Here's how the part is built. I have some questions about the finished solid (model axes, mm). Face numbers are marked on the shaded views. A direction names the side the tool comes from. Round coordinates to 2 decimals unless told otherwise and drop trailing zeros. Write each loop counter-clockwise with the first axis right and the second up, starting at its lowest first coordinate (ties: lowest second). Pieces come first, ordered by that corner, then holes. Notation, with made-up numbers: (85.5, 64) -> (97.5, 64) arc R18 ccw to (97.5, 87) -> close; hole circle Ø9 at (32.5, 4). An arc over 180 degrees is marked (long way). Put each result on its own line as item: value. Start each with the question number.
1) I want a section at A-A, the plane y = 16.5. List the corners of the cut face in (x, z) for me, then the cut area to 3 significant figures.
2) I want a section at C-C, the plane x = 10.5. List the corners of the cut face in (y, z) for me, then the cut area to 3 significant figures.
3) I want a section at D-D, the plane z = 4.75. List the corners of the cut face in (x, y) for me.
4) Will these pins go through, and if not, where does the flat tip stop? P1, Ø0.6, axis at y = 3, z = 10.5, coming from the +X side; P2, Ø3, axis at x = 34, z = 8.5, coming from the -Y side; P3, Ø8, axis at x = 36, y = 10, coming from the +Z side; P4, Ø4, axis at x = 19.5, y = 5, coming from the +Z side.
5) We'd pull the mould along Z, two halves only. Please class the marked faces 4, 5 and 6: released by +Z, released by -Z, zero draft, split by the parting line, or undercut.
6) If I drill on line 1 along Y through (x, z) = (22, 0.2); line 2 along Z through (x, y) = (23, 31.5); line 3 along Z through (x, y) = (24, 13), over which ranges is the centre line in solid material (lowest first)? Write a range as [from, to].
7) I want a section at B-B, the plane x = 33. List the corners of the cut face in (y, z) for me, then the cut area to 3 significant figures.
8) Which directions (+Z, -Z, +X, -X, +Y, -Y) give clear straight access to the entire face, cutting with the end or side of a thin tool? Please do the marked faces 1, 2 and 3.
Autodesk Inventor part; units mm, degrees
ref_plane "YZ Plane" through (0, 0, 0) normal (1, 0, 0) x (0, 1, 0)
ref_plane "XZ Plane" through (0, 0, 0) normal (0, 1, 0) x (-1, 0, 0)
ref_plane "XY Plane" through (0, 0, 0) normal (0, 0, 1) x (1, 0, 0)
sketch "Sketch1" plane through (0, 0, 0) normal (0, 0, 1) x (1, 0, 0)
  line L0 (0, 0) -> (44, 0)
  line L1 (44, 0) -> (44, 33)
  line L2 (44, 33) -> (0, 33)
  line L3 (0, 33) -> (0, 0)
  line L4 (2, 1.5) -> (44, 1.5)
  line L5 (44, 1.5) -> (44, 31.5)
  line L6 (44, 31.5) -> (2, 31.5)
  line L7 (2, 31.5) -> (2, 1.5)
  dimension "d0" = 44
  dimension "d1" = 33
  dimension "d2" = 42
  dimension "d3" = 30
  dimension "d4" = 2
  dimension "d5" = 0
  dimension "d6" = 1.5
extrude "Extrusion1" add sketch "Sketch1" along normal blind 11
shell "Shell1" thickness 1.25 removed faces 1 at (44, 11, 3.6667)
sketch "Sketch2" plane through (0, 0, 11) normal (0, 0, 1) x (1, 0, 0)
  circle A0 centre (22, 16.5) radius 8
  circle A1 centre (22, 16.5) radius 8.75
  point P0 (0, 0)
  dimension "d10" = 16
  dimension "d11" = 17.5
extrude "Extrusion2" add sketch "Sketch2" along normal blind 1.5
sketch "Sketch3" plane through (22, 16.5, 11) normal (0, 0, 1) x (1, 0, 0)
  line L0 (1.47, 5.1769) -> (11.6334, 5.1769)
  line L1 (11.6334, 5.1769) -> (11.6334, -5.2059)
  line L2 (11.6334, -5.2059) -> (1.47, -5.2059)
  line L3 (1.47, -5.2059) -> (1.47, 5.1769)
  line L4 (1.47, 5.1769) -> (11.6334, -5.2059) construction
  line L5 (11.6334, 5.1769) -> (1.47, -5.2059) construction
  point P0 (-22, -16.5)
  point P1 (6.5517, -0.0145)
extrude "Extrusion3" cut sketch "Sketch2" against normal blind 0.6 contours A0
sketch "Sketch4" plane through (0, 0, 0) normal (0, 0, -1) x (-1, 0, 0)
  circle A0 centre (-22, 16.5) radius 8.7
  line L0 (-44, 33) -> (0, 33)
  line L1 (0, 33) -> (0, 0)
  dimension "d16" = 17.4
  dimension "d22" = 16.5
  dimension "d23" = 22
extrude "Extrusion4" cut sketch "Sketch4" against normal blind 0.6
chamfer "Chamfer1" distance 1.5 angle 45 1 edges at (13.25, 16.5, 11)
extrude "Extrusion5" cut sketch "Sketch3" along normal blind 2
sketch "Sketch5" plane through (0, 33, 0) normal (0, 1, 0) x (1, 0, 0)
  line L0 (0, 0) -> (3, 0)
  line L1 (3, 0) -> (3, -3)
  line L2 (3, -3) -> (0, -3)
  line L3 (0, -3) -> (0, 0)
  line L4 (0, 0) -> (44, 0)
  line L5 (44, 0) -> (41, 0)
  line L6 (41, 0) -> (41, -3)
  line L7 (41, -3) -> (44, -3)
  line L8 (44, -3) -> (44, 0)
  dimension "d26" = 3
  dimension "d27" = 3
  dimension "d28" = 3
  dimension "d29" = 3
extrude "Extrusion6" cut sketch "Sketch5" against normal through all
sketch "Sketch6" plane through (0, 0, 11) normal (-1, 0, 0) x (0, 0, 1)
  line L0 (0, 0) -> (0, 33)
  line L1 (-11, 33) -> (-11, 0)
  line L2 (0, 0) -> (-11, 0)
  line L3 (-11, 0) -> (-11, 33)
  line L4 (-11, 33) -> (0, 33)
  line L5 (0, 33) -> (0, 0)
extrude "Extrusion7" cut sketch "Sketch6" against normal blind 0.25
chamfer "Chamfer2" distance 3 angle 45 2 edges at (3, 16.5, 0) (41, 16.5, 0)
sketch "Sketch7" plane through (0, 0, 11) normal (0, 0, 1) x (1, 0, 0)
  line L0 (44, 1.25) -> (44, 31.75)
  line L1 (44, 28) -> (29, 28)
  line L2 (29, 28) -> (29, 25)
  line L3 (29, 25) -> (44, 25)
  line L4 (44, 25) -> (44, 28)
  line L5 (44, 33) -> (0.25, 33)
  line L6 (44, 28.5) -> (29, 28.5)
  line L7 (29, 28.5) -> (29, 24.5)
  line L8 (29, 24.5) -> (44, 24.5)
  line L9 (44, 24.5) -> (44, 28.5)
  point P0 (0, 0)
  dimension "d37" = 15
  dimension "d38" = 3
  dimension "d39" = 5
  dimension "d40" = 4
extrude "Extrusion8" cut sketch "Sketch7" against normal blind 1.5 contours L8 L7 L3 L0 | L1 L7 L6 L0
sketch "Sketch8" plane through (44, 1.25, 9.75) normal (0, 0, -1) x (-1, 0, 0)
  line L0 (0, 26.75) -> (15, 26.75)
  line L1 (0, 23.75) -> (15, 23.75)
  line L2 (0, 26.75) -> (4.5, 26.75)
  line L3 (4.5, 26.75) -> (4.5, 23.75)
  line L4 (4.5, 23.75) -> (0, 23.75)
  line L5 (0, 23.75) -> (0, 26.75)
  point P0 (44, -1.25)
  point P1 (4.5, 26.75)
  dimension "d43" = 4.5
extrude "Extrusion9" add sketch "Sketch8" along normal blind 2.5
chamfer "Chamfer3" distance 2.25 angle 45 2 edges at (44, 26.5, 7.25) (39.5, 26.5, 7.25)
pattern_linear "Rectangular Pattern1" count 2 spacing 20 along (0, -1, 0) of "Extrusion9", "Chamfer3", "Extrusion8"
sketch "Sketch9" plane through (0, 0, 11) normal (0, 0, 1) x (1, 0, 0)
  line L0 (44, 4.5) -> (29, 4.5)
  line L1 (4.75, 1.25) -> (39.25, 1.25)
  line L2 (44, 4.5) -> (39.25, 4.5)
  line L3 (39.25, 4.5) -> (39.25, 1.25)
  line L4 (39.25, 1.25) -> (44, 1.25)
  line L5 (44, 1.25) -> (44, 4.5)
  point P0 (0, 0)
extrude "Extrusion10" cut sketch "Sketch9" against normal blind 2.5
properties part number "ButtonBatteryHolder"
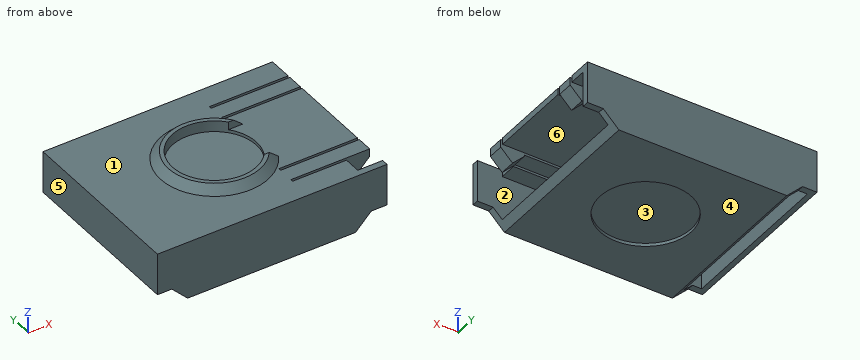
Findings:
1. outline: (0.25, 3) -> (1.25, 3) -> (1.25, 9.75) -> (44, 9.75) -> (44, 11) -> (30, 11) -> (30, 10.4) -> (14, 10.4) -> (14, 12.5) -> (13.25, 12.5) -> (11.75, 11) -> (0.25, 11) -> close; (4.75, 1.25) -> (6, 0) -> (13.3, 0) -> (13.3, 0.6) -> (30.7, 0.6) -> (30.7, 0) -> (38, 0) -> (39.25, 1.25) -> close
1. area: 85.2 mm2
2. outline: (0, 0) -> (33, 0) -> (33, 11) -> (0, 11) -> close; hole (1.25, 1.25) -> (31.75, 1.25) -> (31.75, 9.75) -> (1.25, 9.75) -> close
2. area: 104 mm2
3. outline: (0.25, 0) -> (44, 0) -> (44, 1.25) -> (1.25, 1.25) -> (1.25, 31.75) -> (44, 31.75) -> (44, 33) -> (0.25, 33) -> close
4. P1: stops at x = 39.25
4. P2: stops at y = 0
4. P3: stops at z = 11
4. P4: stops at z = 11.48
5. face 4: released by -Z
5. face 5: zero draft
5. face 6: undercut
6. line 1: y = [0, 7.8], [25.2, 33]
6. line 2: z = [0, 1.25], [9.75, 11]
6. line 3: z = [0.6, 1.25], [9.75, 10.4]
7. outline: (0, 0) -> (33, 0) -> (33, 11) -> (28.5, 11) -> (28.5, 9.75) -> (31.75, 9.75) -> (31.75, 1.25) -> (1.25, 1.25) -> (1.25, 9.75) -> (4.5, 9.75) -> (4.5, 11) -> (0, 11) -> close; (5, 9.75) -> (8, 9.75) -> (8, 11) -> (5, 11) -> close; (8.5, 9.75) -> (24.5, 9.75) -> (24.5, 11) -> (8.5, 11) -> close; (25, 9.75) -> (28, 9.75) -> (28, 11) -> (25, 11) -> close
7. area: 101 mm2
8. face 1: +Z
8. face 2: +X
8. face 3: -Z
